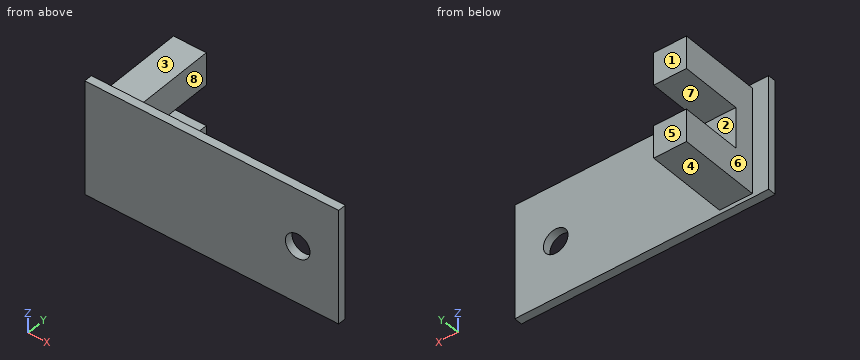
```python
from build123d import *

# Parameters (mm, degrees)
SKETCH1_W           = 31
SKETCH1_H           = 14
BOSS_EXTRUDE1_DEPTH = 1
SKETCH2_W           = 4
SKETCH2_H           = 4
BOSS_EXTRUDE2_DEPTH = 10
SKETCH3_R           = 1.5
CUT_EXTRUDE1_DEPTH  = 36.454195802
SKETCH4_W           = 4
SKETCH4_H           = 5
BOSS_EXTRUDE3_DEPTH = 2.5


with BuildPart() as part:
    # Sketch1 → Boss-Extrude1 (new body)
    with BuildSketch(Plane(origin=(0, 0, 0), x_dir=(1, 0, 0), z_dir=(0, 1, 0))):
        with Locations((15.5, -7)):
            Rectangle(SKETCH1_W, SKETCH1_H)
    extrude(amount=BOSS_EXTRUDE1_DEPTH)

    # Sketch2 → Boss-Extrude2 (add)
    with BuildSketch(Plane(origin=(0, 1, 0), x_dir=(1, 0, 0), z_dir=(0, 1, 0))):
        with Locations((4, -11.5)):
            Rectangle(SKETCH2_W, SKETCH2_H)
        with Locations((4, -2.5)):
            Rectangle(SKETCH2_W, SKETCH2_H)
    extrude(amount=BOSS_EXTRUDE2_DEPTH)

    # Sketch3 → Cut-Extrude1 (cut, through all)
    with BuildSketch(Plane(origin=(0, 1, 0), x_dir=(1, 0, 0), z_dir=(0, 1, 0))):
        with Locations(Location((26, -7, 0), (0, 0, 270))):
            Circle(SKETCH3_R)
    extrude(amount=-CUT_EXTRUDE1_DEPTH, mode=Mode.SUBTRACT)

    # Sketch4 → Boss-Extrude3 (add)
    with BuildSketch(Plane(origin=(0, 1, 0), x_dir=(1, 0, 0), z_dir=(0, 1, 0))):
        with Locations((4, -7)):
            Rectangle(SKETCH4_W, SKETCH4_H)
    extrude(amount=BOSS_EXTRUDE3_DEPTH)


solid = part.part
```
Design review of the part built by this model. Coordinates are the model's own, in mm. Face numbers are marked on the shaded views. A direction names the side the tool comes from. Coordinates: 2 decimals unless noted, no trailing zeros. Order: outer loops, then holes, each group sorted by start corner. A loop starts at its lowest first (then second) coordinate and runs counter-clockwise, first axis right, second up. Notation, with made-up numbers: M 88,75.25 L 95,75.25 A9 cw 95,80.25 Z; hole C 34.5,-36.75 d9. An arc over 180 degrees is marked long. Answer as a JSON object with one key per item and string values. Group by question number.
1) Add section D-D, the plane z = 3.5. Write out the cut boundary in (x, y).
2) Mouldability with a two-part tool opening along Z and no side actions: class the marked faces 1, 2 and 3 as pulls with the +Z half, pulls with the -Z half, needs draft (parallel to the pull), parting line crosses it, or undercut.
3) Wall thickness on L1, parallel to X at y = 0.2, z = 7; L2, parallel to Y at x = 27.5, z = 9.5; L3, parallel to X at y = 6, z = 9.75: over which ranges is each line inside the solid? List them lowest first.
4) For pin 1 (2 mm diameter, centred on x = 4, z = 6, fed in from +Y); pin 2 (1 mm diameter, centred on y = 4.5, z = 12.5, fed in from +X); pin 3 (3 mm diameter, centred on x = 3.5, y = 4.5, fed in from +Z); pin 4 (1 mm diameter, centred on x = 9.5, z = 10, fed in from -Y), all flat-tipped, find the tip position at first contact; note any pin that passes through.
5) Add section A-A, the plane x = 26. Write out the cut boundary in (y, z).
6) Add section B-B, the plane y = 7. Write out the cut boundary in (x, z), then the cut area to 3 significant figures.
7) Tool access review of the marked faces 4, 5, 6, 7 and 8: name each direction out of +Z, -Z, +X, -X, +Y, -Y from which nothing blocks a thin tool from reaching the whole face with its end or side.
8) Add section C-C, the plane z = 7. Write out the cut boundary in (x, y).
Computed values:
{
 "1": {"outline": "M 0,0 L 31,0 L 31,1 L 6,1 L 6,11 L 2,11 L 2,1 L 0,1 Z"},
 "2": {"face 1": "needs draft", "face 2": "undercut", "face 3": "pulls with the +Z half"},
 "3": {"L1": "x = 0 to 24.5, 27.5 to 31", "L2": "y = 0 to 1", "L3": "x = 2 to 6"},
 "4": {"pin 1": "stops at y = 3.5", "pin 2": "stops at x = 6", "pin 3": "stops at z = 13.5", "pin 4": "stops at y = 0"},
 "5": {"outline": "M 0,0 L 1,0 L 1,5.5 L 0,5.5 Z; M 0,8.5 L 1,8.5 L 1,14 L 0,14 Z"},
 "6": {"outline": "M 2,0.5 L 6,0.5 L 6,4.5 L 2,4.5 Z; M 2,9.5 L 6,9.5 L 6,13.5 L 2,13.5 Z", "area": "32.0 mm^2"},
 "7": {"face 4": "-Z, +X, -X, +Y", "face 5": "+Z, -Z, +X, -X, +Y", "face 6": "+Z, -Z, -X, +Y", "face 7": "+X, -X, +Y", "face 8": "+Z, -Z, +X, +Y"},
 "8": {"outline": "M 0,0 L 24.5,0 L 24.5,1 L 6,1 L 6,3.5 L 2,3.5 L 2,1 L 0,1 Z; M 27.5,0 L 31,0 L 31,1 L 27.5,1 Z"}
}
